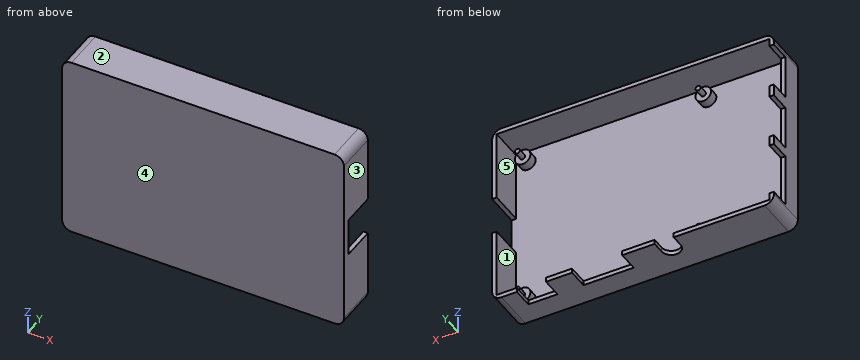
```python
from build123d import *

# Parameters (mm, degrees)
CROQUIS1_W              = 89
CROQUIS1_H              = 60
SALIENTE_EXTRUIR1_DEPTH = 2.5
CROQUIS2_R              = 2.5
SALIENTE_EXTRUIR2_DEPTH = 3
CROQUIS3_R              = 0.83
SALIENTE_EXTRUIR3_DEPTH = 3
CROQUIS4_W              = 89
CROQUIS4_H              = 1.45
SALIENTE_EXTRUIR4_DEPTH = 11.1
CROQUIS5_W              = 1.45
CROQUIS5_H              = 60
SALIENTE_EXTRUIR5_DEPTH = 13.6
CORTAR_EXTRUIR1_REACH   = 62
CORTAR_EXTRUIR2_REACH   = 62
CROQUIS7_W              = 16.1
CROQUIS7_H              = 6.5
CORTAR_EXTRUIR3_REACH   = 62
CROQUIS8_W              = 9.32
CROQUIS8_H              = 6.5
REDONDEO1_R             = 3
CROQUIS12_W             = 1.45
CROQUIS12_H             = 57.1
SALIENTE_EXTRUIR7_DEPTH = 11.1
CORTAR_EXTRUIR5_REACH   = 92.45
CROQUIS13_W             = 17
CROQUIS13_H             = 6.5
CORTAR_EXTRUIR6_REACH   = 92.45
CROQUIS14_W             = 14.2
CROQUIS14_H             = 6.5
REDONDEO2_R             = 3
CROQUIS15_W             = 1.45
CROQUIS15_H             = 12.1
CORTAR_EXTRUIR7_DEPTH   = 11.1


with BuildPart() as part:
    # Croquis1 → Saliente-Extruir1 (new body)
    with BuildSketch(Plane(origin=(0, 0, 0), x_dir=(1, 0, 0), z_dir=(0, 1, 0))):
        Rectangle(CROQUIS1_W, CROQUIS1_H)
    extrude(amount=-SALIENTE_EXTRUIR1_DEPTH)

    # Croquis2 → Saliente-Extruir2 (add)
    with BuildSketch(Plane(origin=(0, 0, 0), x_dir=(1, 0, 0), z_dir=(0, 1, 0))):
        with Locations((40.75, 24.5)):
            Circle(CROQUIS2_R)
        with Locations((40.75, -24.5)):
            Circle(CROQUIS2_R)
        with Locations((-17.25, 24.5)):
            Circle(CROQUIS2_R)
        with Locations((-17.25, -24.5)):
            Circle(CROQUIS2_R)
    extrude(amount=SALIENTE_EXTRUIR2_DEPTH)

    # Croquis3 → Saliente-Extruir3 (add)
    with BuildSketch(Plane(origin=(0, 3, 0), x_dir=(1, 0, 0), z_dir=(0, 1, 0))):
        with Locations((-17.25, 24.5)):
            Circle(CROQUIS3_R)
        with Locations((40.75, 24.5)):
            Circle(CROQUIS3_R)
        with Locations((40.75, -24.5)):
            Circle(CROQUIS3_R)
        with Locations((-17.25, -24.5)):
            Circle(CROQUIS3_R)
    extrude(amount=SALIENTE_EXTRUIR3_DEPTH)

    # Croquis4 → Saliente-Extruir4 (add)
    with BuildSketch(Plane(origin=(0, 0, 0), x_dir=(1, 0, 0), z_dir=(0, 1, 0))):
        with Locations((0, -29.275)):
            Rectangle(CROQUIS4_W, CROQUIS4_H)
        with Locations((0, 29.275)):
            Rectangle(CROQUIS4_W, CROQUIS4_H)
    extrude(amount=SALIENTE_EXTRUIR4_DEPTH)

    # Croquis5 → Saliente-Extruir5 (add)
    with BuildSketch(Plane.XZ.offset(2.5)):
        with Locations((45.225, 0)):
            Rectangle(CROQUIS5_W, CROQUIS5_H)
    extrude(amount=-SALIENTE_EXTRUIR5_DEPTH)

    # Croquis6 → Cortar-Extruir1 (cut, up to next)
    with BuildSketch(Plane(origin=(0, 0, -30), x_dir=(-1, 0, 0), z_dir=(0, 0, -1)), mode=Mode.PRIVATE) as cortar_extruir1_sk1:
        with BuildLine():
            Line((6.2, 7.1), (6.2, 11.1))
            Line((6.2, 11.1), (12.3, 11.1))
            Line((12.3, 11.1), (12.3, 7.1))
            ThreePointArc((12.3, 7.1), (9.25, 4.05), (6.2, 7.1))
        make_face()
    cortar_extruir1_tool1 = extrude(cortar_extruir1_sk1.sketch, amount=-CORTAR_EXTRUIR1_REACH, mode=Mode.PRIVATE) & part.part
    add(cortar_extruir1_tool1.solids().sort_by_distance((-9.25, 7.866038, -30))[0], mode=Mode.SUBTRACT)

    # Croquis7 → Cortar-Extruir2 (cut, up to next)
    with BuildSketch(Plane(origin=(0, 0, -30), x_dir=(-1, 0, 0), z_dir=(0, 0, -1)), mode=Mode.PRIVATE) as cortar_extruir2_sk1:
        with Locations((-12.25, 7.85)):
            Rectangle(CROQUIS7_W, CROQUIS7_H)
    cortar_extruir2_tool1 = extrude(cortar_extruir2_sk1.sketch, amount=-CORTAR_EXTRUIR2_REACH, mode=Mode.PRIVATE) & part.part
    add(cortar_extruir2_tool1.solids().sort_by_distance((12.25, 7.85, -30))[0], mode=Mode.SUBTRACT)

    # Croquis8 → Cortar-Extruir3 (cut, up to next)
    with BuildSketch(Plane(origin=(0, 0, -30), x_dir=(-1, 0, 0), z_dir=(0, 0, -1)), mode=Mode.PRIVATE) as cortar_extruir3_sk1:
        with Locations((-33.34, 7.85)):
            Rectangle(CROQUIS8_W, CROQUIS8_H)
    cortar_extruir3_tool1 = extrude(cortar_extruir3_sk1.sketch, amount=-CORTAR_EXTRUIR3_REACH, mode=Mode.PRIVATE) & part.part
    add(cortar_extruir3_tool1.solids().sort_by_distance((33.34, 7.85, -30))[0], mode=Mode.SUBTRACT)

    # Redondeo1
    redondeo1_edges = [part.edges().sort_by_distance(p)[0] for p in [
        (45.95, 4.3, 30),
        (45.95, 4.3, -30),
    ]]
    fillet(redondeo1_edges, radius=REDONDEO1_R)

    # Croquis12 → Saliente-Extruir7 (add)
    with BuildSketch(Plane(origin=(0, 0, 0), x_dir=(1, 0, 0), z_dir=(0, 1, 0))):
        with Locations((-43.775, 0)):
            Rectangle(CROQUIS12_W, CROQUIS12_H)
    extrude(amount=SALIENTE_EXTRUIR7_DEPTH)

    # Croquis13 → Cortar-Extruir5 (cut, up to next)
    with BuildSketch(Plane.ZY.offset(44.5), mode=Mode.PRIVATE) as cortar_extruir5_sk1:
        with Locations((-17.75, 7.85)):
            Rectangle(CROQUIS13_W, CROQUIS13_H)
    cortar_extruir5_tool1 = extrude(cortar_extruir5_sk1.sketch, amount=-CORTAR_EXTRUIR5_REACH, mode=Mode.PRIVATE) & part.part
    add(cortar_extruir5_tool1.solids().sort_by_distance((-44.5, 7.85, -17.75))[0], mode=Mode.SUBTRACT)

    # Croquis14 → Cortar-Extruir6 (cut, up to next)
    with BuildSketch(Plane.ZY.offset(44.5), mode=Mode.PRIVATE) as cortar_extruir6_sk1:
        with Locations((0.95, 7.85)):
            Rectangle(CROQUIS14_W, CROQUIS14_H)
    cortar_extruir6_tool1 = extrude(cortar_extruir6_sk1.sketch, amount=-CORTAR_EXTRUIR6_REACH, mode=Mode.PRIVATE) & part.part
    add(cortar_extruir6_tool1.solids().sort_by_distance((-44.5, 7.85, 0.95))[0], mode=Mode.SUBTRACT)
    # Croquis14 → Cortar-Extruir6 (cut, up to next)
    with BuildSketch(Plane.ZY.offset(44.5), mode=Mode.PRIVATE) as cortar_extruir6_sk2:
        with Locations((18.95, 7.85)):
            Rectangle(CROQUIS14_W, CROQUIS14_H)
    cortar_extruir6_tool2 = extrude(cortar_extruir6_sk2.sketch, amount=-CORTAR_EXTRUIR6_REACH, mode=Mode.PRIVATE) & part.part
    add(cortar_extruir6_tool2.solids().sort_by_distance((-44.5, 7.85, 18.95))[0], mode=Mode.SUBTRACT)

    # Redondeo2
    redondeo2_edges = [part.edges().sort_by_distance(p)[0] for p in [
        (-44.5, 4.3, 30),
        (-44.5, 4.3, -30),
    ]]
    fillet(redondeo2_edges, radius=REDONDEO2_R)

    # Croquis15 → Cortar-Extruir7 (cut)
    with BuildSketch(Plane(origin=(0, 11.1, 0), x_dir=(1, 0, 0), z_dir=(0, 1, 0))):
        with Locations((45.225, 0)):
            Rectangle(CROQUIS15_W, CROQUIS15_H)
    extrude(amount=-CORTAR_EXTRUIR7_DEPTH, mode=Mode.SUBTRACT)


solid = part.part
```
Input: part model. Units: mm. Frame: model coordinates. Face numbers are marked on the shaded views. A direction names the side the tool comes from. Give positions to 0.01 mm unless a question says otherwise; leave off trailing zeros. Loops run counter-clockwise (first coordinate to the right, second up) from the corner with the lowest first, then second, coordinate; pieces in that order, holes last. Notation, with made-up numbers: M -9.5,83.25 L 44.5,83.25 A28 ccw 44.5,119.25 Z; hole C 70,44.5 d4. An arc over 180 degrees is marked long. Answer as CSV lines item,"result". Start each with the question number.
1. Section C-C on z = -2. Return loops of the section in (x, y), plus the area to 3 significant figures.
2. Section B-B on x = -2. Return loops of the section in (y, z), plus the area to 3 significant figures.
3. Section A-A on z = -8. Return loops of the section in (x, y), plus the area to 3 significant figures.
4. Line query: L1, parallel to X at y = 3, z = -14; L2, parallel to X at y = 1.5, z = 24.5; L3, parallel to Z at x = -35, y = 4. Output: solid intervals per line, ascending.
5. Pin query (flat end, axial travel): P1, Ø0.7, axis at y = 7, z = -29, coming from the +X side; P2, Ø1.2, axis at x = -43.5, z = -0.5, coming from the +Y side; P3, Ø1.5, axis at x = -16.5, z = -10, coming from the +Y side. Return the tip coordinate at first contact, or that it passes through.
6. Pull-direction query (X, two-part tool) for the marked faces 3, 4 and 5; classes: released by +X, released by -X, zero draft, split by the parting line, or undercut.
7. Reachability of the marked faces 1 and 2 from +Z, -Z, +X, -X, +Y, -Y: full face, straight path, thin tool, end or side. Return the list, or none.
Computed values:
1,outline,"M -44.5,-2.5 L 45.95,-2.5 L 45.95,0 L -43.05,0 L -43.05,4.6 L -44.5,4.6 Z"
1,area,"233 mm²"
2,outline,"M -2.5,-30 L 11.1,-30 L 11.1,-28.55 L 0,-28.55 L 0,28.55 L 11.1,28.55 L 11.1,30 L -2.5,30 Z"
2,area,"182 mm²"
3,outline,"M -44.5,-2.5 L 45.95,-2.5 L 45.95,11.1 L 44.5,11.1 L 44.5,0 L -43.05,0 L -43.05,11.1 L -44.5,11.1 Z"
3,area,"258 mm²"
4,L1,"x = -44.5 to -43.05, 44.5 to 45.95"
4,L2,"x = -44.5 to -43.05, -19.75 to -14.75, 38.25 to 43.25, 44.5 to 45.95"
4,L3,"z = -30 to -28.55, 28.55 to 30"
5,P1,"stops at x = 45.46"
5,P2,"stops at y = 4.6"
5,P3,"stops at y = 0"
6,face 3,"released by +X"
6,face 4,"zero draft"
6,face 5,"undercut"
7,face 1,"+Y"
7,face 2,"+Z, +X, -X, +Y, -Y"
